Geometry: final body of the model. Coordinates: model frame, mm. A direction names the side the tool comes from. Give positions to 0.01 mm unless a question says otherwise; leave off trailing zeros. Write each loop counter-clockwise with the first axis right and the second up, starting at its lowest first coordinate (ties: lowest second). Pieces come first, ordered by that corner, then holes. Notation, with made-up numbers: (-10, 71) -> (9, 71) arc R14 cw to (9, 78) -> close; hole circle Ø3 at (54, 27.25). An arc over 180 degrees is marked (long way). Answer in a Markdown table with one row per item. Add a question column.
Item 1: Material intervals for probe 1 along Y at (x, z) = (0, 5.05); probe 2 along X at (y, z) = (7.5, -6.35); probe 3 along Z at (x, y) = (2.75, 9.25), sorted ascending. Write a range as from..to.
Item 2: First-contact query: P1, Ø0.9, axis at x = 0, y = -2, coming from the -Z side; P2, Ø3, axis at y = 6, z = 5.5, coming from the -X side; P3, Ø4, axis at y = 9.5, z = 5, coming from the -X side. Flat tips, straight axial feed; report the tip coordinate or a pass-through.
Item 3: Section query A-A on x = 0. State how many separate pieces and enclosed holes the cut face has, plus the area to 3 significant figures.
Item 4: Access query for faces 1 (the flat face through (0, -2, -1.95)), 2 (the flat face through (1.95, -2, 0)), 3 (the flat face through (3.75, 6, 6)), 4 (the flat face through (-3.75, 3, 0)). Directions: +Z, -Z, +X, -X, +Y, -Y. A direction counts if a zero-diameter tool reaches every point of the face in a straight line with its end or side. Return the directions, or none.
Item 5: Section query B-B on z = 5.25. Output: boundary loops of the cut face in (x, y), plus the area to 3 significant figures.
Item 6: Draft query along Y for faces 5 (the flat face through (-3.75, 6, -6)), 6 (the cylindrical face through (0.08, 11.25, 5.5)), 7 (the cylindrical face through (1.78, -1.09, -0.03)). Return one class per face: +Y half, -Y half, draft (parallel to the pull), parting line (faces both ways), or undercut.
Item 7: Section query C-C on z = 3.5. Output: boundary loops of the cut face in (x, y).
```python
from build123d import *

# Parameters (mm, degrees)
EXTRUDE_1_DEPTH                 = 7.5
EXTRUDE_1_DEPTH_BACK            = 7.5
SKETCH_1_R                      = 2.75
CUT_EXTRUDE_1_DEPTH             = 3.75
CUT_EXTRUDE_1_DEPTH_BACK        = 3.75
SKETCH_2_W                      = 7.5
SKETCH_2_H                      = 8.25
SKETCH_3_W                      = 7.5
SKETCH_3_H                      = 7.5
CUT_EXTRUDE_2_DEPTH             = 2
SKETCH_4_W                      = 3
SKETCH_4_H                      = 3
EXTRUDE_2_DEPTH                 = 1
EXTRUDE_3_DEPTH                 = 2
EXTRUDE_3_DEPTH_BACK            = 2
CUT_EXTRUDE_3_REACH             = 17.462
CUT_EXTRUDE_3_DIRECTION_2_REACH = 17.462
FILLET_1_R                      = 0.1
FILLET_2_R                      = 0.2


with BuildPart() as part:
    # 草图1 → 凸台-拉伸1 (new, two sides: drawn at the far end of the back side and taken through both)
    with BuildSketch(Plane.XY.offset(-EXTRUDE_1_DEPTH_BACK)):
        with BuildLine():
            Line((-7.5, 0), (7.5, 0))
            Line((7.5, 0), (3.75, 3.75))
            Line((3.75, 3.75), (3.75, 7.5))
            ThreePointArc((3.75, 7.5), (0, 11.25), (-3.75, 7.5))
            Line((-3.75, 7.5), (-3.75, 3.75))
            Line((-3.75, 3.75), (-7.5, 0))
        make_face()
        with Locations((0, 7.5)):
            Circle(SKETCH_1_R, mode=Mode.SUBTRACT)
    extrude(amount=EXTRUDE_1_DEPTH + EXTRUDE_1_DEPTH_BACK)

    # 草图2 → 切除-拉伸1 (cut, two sides: drawn at the far end of the back side and taken through both)
    with BuildSketch(Plane.XY.offset(-CUT_EXTRUDE_1_DEPTH_BACK)):
        with Locations((0, 7.875)):
            Rectangle(SKETCH_2_W, SKETCH_2_H)
    extrude(amount=CUT_EXTRUDE_1_DEPTH + CUT_EXTRUDE_1_DEPTH_BACK, mode=Mode.SUBTRACT)

    # 草图3 → 切除-拉伸2 (cut)
    with BuildSketch(Plane(origin=(0, 3.75, 0), x_dir=(-1, 0, 0), z_dir=(0, 1, 0))):
        Rectangle(SKETCH_3_W, SKETCH_3_H)
    extrude(amount=-CUT_EXTRUDE_2_DEPTH, mode=Mode.SUBTRACT)

    # 草图4 → 凸台-拉伸2 (add)
    with BuildSketch(Plane.XZ):
        Rectangle(SKETCH_4_W, SKETCH_4_H)
    extrude(amount=EXTRUDE_2_DEPTH)

    # 草图5 → 凸台-拉伸3 (add, two sides: drawn at the far end of the back side and taken through both)
    with BuildSketch(Plane.XY.offset(-EXTRUDE_3_DEPTH_BACK)):
        with BuildLine():
            Line((-1.95, -2.5), (1.95, -2.5))
            Line((1.95, -2.5), (1.95, -1.555590279))
            ThreePointArc((1.95, -1.555590279), (1.780042303, -1.088161527), (1.5, -0.677124344))
            Line((1.5, -0.677124344), (-1.5, -0.677124344))
            ThreePointArc((-1.5, -0.677124344), (-1.780042303, -1.088161527), (-1.95, -1.555590279))
            Line((-1.95, -1.555590279), (-1.95, -2.5))
        make_face()
    extrude(amount=EXTRUDE_3_DEPTH + EXTRUDE_3_DEPTH_BACK)

    # 草图6 → 切除-拉伸3 (cut, up to next)
    with BuildSketch(Plane(origin=(0, 0, 0), x_dir=(0, 0, -1), z_dir=(1, 0, 0)), mode=Mode.PRIVATE) as cut_extrude_3_sk1:
        with BuildLine():
            Line((1.95, -2.5), (1.95, -1.555590279))
            ThreePointArc((1.95, -1.555590279), (1.780042303, -1.088161527), (1.5, -0.677124344))
            Line((1.5, -0.677124344), (2, -0.677124344))
            Line((2, -0.677124344), (2, -2.5))
            Line((2, -2.5), (1.95, -2.5))
        make_face()
    cut_extrude_3_tool1 = extrude(cut_extrude_3_sk1.sketch, amount=-CUT_EXTRUDE_3_REACH, mode=Mode.PRIVATE) & part.part
    # 草图6 → 切除-拉伸3 (cut, up to next)
    with BuildSketch(Plane(origin=(0, 0, 0), x_dir=(0, 0, -1), z_dir=(1, 0, 0)), mode=Mode.PRIVATE) as cut_extrude_3_sk2:
        with BuildLine():
            Line((-2, -2.5), (-2, -0.677124344))
            Line((-2, -0.677124344), (-1.5, -0.677124344))
            ThreePointArc((-1.5, -0.677124344), (-1.780042303, -1.088161527), (-1.95, -1.555590279))
            Line((-1.95, -1.555590279), (-1.95, -2.5))
            Line((-1.95, -2.5), (-2, -2.5))
        make_face()
    cut_extrude_3_tool2 = extrude(cut_extrude_3_sk2.sketch, amount=-CUT_EXTRUDE_3_REACH, mode=Mode.PRIVATE) & part.part
    add(cut_extrude_3_tool1.solids().sort_by_distance((0, -1.175075, -1.873038))[0], mode=Mode.SUBTRACT)
    add(cut_extrude_3_tool2.solids().sort_by_distance((0, -1.175075, 1.873038))[0], mode=Mode.SUBTRACT)

    # 草图6 → 切除-拉伸3 direction 2 (cut, up to next)
    with BuildSketch(Plane(origin=(0, 0, 0), x_dir=(0, 0, -1), z_dir=(1, 0, 0)), mode=Mode.PRIVATE) as cut_extrude_3_direction_2_sk1:
        with BuildLine():
            Line((1.95, -2.5), (1.95, -1.555590279))
            ThreePointArc((1.95, -1.555590279), (1.780042303, -1.088161527), (1.5, -0.677124344))
            Line((1.5, -0.677124344), (2, -0.677124344))
            Line((2, -0.677124344), (2, -2.5))
            Line((2, -2.5), (1.95, -2.5))
        make_face()
    cut_extrude_3_direction_2_tool1 = extrude(cut_extrude_3_direction_2_sk1.sketch, amount=CUT_EXTRUDE_3_DIRECTION_2_REACH, mode=Mode.PRIVATE) & part.part
    # 草图6 → 切除-拉伸3 direction 2 (cut, up to next)
    with BuildSketch(Plane(origin=(0, 0, 0), x_dir=(0, 0, -1), z_dir=(1, 0, 0)), mode=Mode.PRIVATE) as cut_extrude_3_direction_2_sk2:
        with BuildLine():
            Line((-2, -2.5), (-2, -0.677124344))
            Line((-2, -0.677124344), (-1.5, -0.677124344))
            ThreePointArc((-1.5, -0.677124344), (-1.780042303, -1.088161527), (-1.95, -1.555590279))
            Line((-1.95, -1.555590279), (-1.95, -2.5))
            Line((-1.95, -2.5), (-2, -2.5))
        make_face()
    cut_extrude_3_direction_2_tool2 = extrude(cut_extrude_3_direction_2_sk2.sketch, amount=CUT_EXTRUDE_3_DIRECTION_2_REACH, mode=Mode.PRIVATE) & part.part
    add(cut_extrude_3_direction_2_tool1.solids().sort_by_distance((0, -1.175075, -1.873038))[0], mode=Mode.SUBTRACT)
    add(cut_extrude_3_direction_2_tool2.solids().sort_by_distance((0, -1.175075, 1.873038))[0], mode=Mode.SUBTRACT)

    # 圆角1
    fillet_1_edges = [part.edges().sort_by_distance(p)[0] for p in [
        (-1.95, -2.5, 0),
        (1.95, -2.5, 0),
        (0, -2.5, -1.95),
        (0, -2.5, 1.95),
    ]]
    fillet(fillet_1_edges, radius=FILLET_1_R)

    # 圆角2
    fillet_2_edges = [part.edges().sort_by_distance(p)[0] for p in [
        (0, 11.25, 7.5),
        (7.5, 0, 0),
        (-7.5, 0, 0),
        (-3.75, 5.625, 7.5),
        (-5.625, 1.875, 7.5),
        (-2.75, 7.5, 7.5),
        (0, 0, 7.5),
        (5.625, 1.875, -7.5),
        (0, 0, -7.5),
        (-5.625, 1.875, -7.5),
        (-3.75, 5.625, -7.5),
        (0, 11.25, -7.5),
        (3.75, 5.625, -7.5),
        (-2.75, 7.5, -7.5),
        (5.625, 1.875, 7.5),
        (3.75, 5.625, 7.5),
    ]]
    fillet(fillet_2_edges, radius=FILLET_2_R)


solid = part.part
```
Findings below:
| question | item | result |
|---|---|---|
| 1 | probe 1 | y = 0..4.75, 10.25..11.25 |
| 1 | probe 2 | x = -3.75..-2.75, 2.75..3.75 |
| 1 | probe 3 | z = -7.5..-3.75, 3.75..7.5 |
| 2 | P1 | stops at z = -1.95 |
| 2 | P2 | stops at x = -3.75 |
| 2 | P3 | stops at x = -3.75 |
| 3 | separate pieces | 3 |
| 3 | enclosed holes | 0 |
| 3 | area | 65.0 mm^2 |
| 4 | face 1 | -Z, +X, -X, -Y |
| 4 | face 2 | +Z, -Z, +X, -Y |
| 4 | face 3 | +Z, -Z, +X, +Y |
| 4 | face 4 | +Y |
| 5 | outline | (-7.16, 0.34) arc R0.2 ccw to (-7.02, 0) -> (7.02, 0) arc R0.2 ccw to (7.16, 0.34) -> (3.75, 3.75) -> (3.75, 7.5) arc R3.75 ccw to (-3.75, 7.5) -> (-3.75, 3.75) -> close; hole circle Ø5.5 at (0, 7.5) |
| 5 | area | 68.5 mm^2 |
| 6 | face 5 | draft |
| 6 | face 6 | +Y half |
| 6 | face 7 | undercut |
| 7 | outline | (-7.16, 0.34) arc R0.2 ccw to (-7.02, 0) -> (7.02, 0) arc R0.2 ccw to (7.16, 0.34) -> (3.75, 3.75) -> (3.75, 1.75) -> (-3.75, 1.75) -> (-3.75, 3.75) -> close |
